Here's how the part is built. I have some questions about the finished solid (model axes, mm). A direction names the side the tool comes from. Give positions to 0.01 mm unless a question says otherwise; leave off trailing zeros. Write each loop counter-clockwise with the first axis right and the second up, starting at its lowest first coordinate (ties: lowest second). Pieces come first, ordered by that corner, then holes. Notation, with made-up numbers: (58, 0) -> (107, 0) arc R16 cw to (107, 17) -> close; hole circle Ø2 at (-17.75, 87). An arc over 180 degrees is marked (long way). Use one line per item in the form item = value.
```python
from build123d import *

# Parameters (mm, degrees)
EXTRUDE_1_DEPTH           = 5
HOLE_WIZARD_M5_1_D        = 5.3
CUT_EXTRUDE_1_DEPTH       = 2.5
HOLE_WIZARD_2_0_2_1_D     = 2
HOLE_WIZARD_2_0_2_1_DEPTH = 5
HOLE_WIZARD_2_0_2_2_D     = 2
HOLE_WIZARD_2_0_2_2_DEPTH = 55
HOLE_WIZARD_M5_2_D        = 5.3
HOLE_WIZARD_M5_2_DEPTH    = 12.4


with BuildPart() as part:
    # 스케치1 → 보스-돌출1 (new, symmetric)
    with BuildSketch(Plane.XY):
        with BuildLine():
            Line((-32, 0), (32, 0))
            Line((32, 0), (32, 6))
            Line((32, 6), (16.781610859, 57.462613925))
            ThreePointArc((16.781610859, 57.462613925), (0, 70), (-16.781610859, 57.462613925))
            Line((-16.781610859, 57.462613925), (-32, 6))
            Line((-32, 6), (-32, 0))
        make_face()
    extrude(amount=EXTRUDE_1_DEPTH, both=True)

    # M5 여유 구멍1 (through all)
    with Locations(Plane.XY.offset(5)):
        with Locations((0, 53)):
            Hole(HOLE_WIZARD_M5_1_D / 2)

    # 스케치4 → 컷-돌출1 (cut)
    with BuildSketch(Plane.XY.offset(5)):
        with BuildLine():
            ThreePointArc((-10.585585486, 60.184777453), (-12.793578355, 53), (-10.585585486, 45.815222547))
            ThreePointArc((-10.585585486, 45.815222547), (-6.418566116, 45.017758083), (-5.621101652, 49.184777453))
            ThreePointArc((-5.621101652, 49.184777453), (-6.793578355, 53), (-5.621101652, 56.815222547))
            ThreePointArc((-5.621101652, 56.815222547), (-6.418566116, 60.982241917), (-10.585585486, 60.184777453))
        make_face()
    cut_extrude_1 = extrude(amount=-CUT_EXTRUDE_1_DEPTH, mode=Mode.SUBTRACT)

    # Ø2.0 (2) 지름 구멍1
    with Locations(Plane.XY.offset(5)):
        with Locations((-8, 53)):
            hole_wizard_2_0_2_1 = Hole(HOLE_WIZARD_2_0_2_1_D / 2, depth=HOLE_WIZARD_2_0_2_1_DEPTH)

    # 대칭 복사1: 컷-돌출1, Ø2.0 (2) 지름 구멍1 across plane
    add(cut_extrude_1.mirror(Plane(origin=(0, 0, 0), x_dir=(0, 0, 1), z_dir=(1, 0, 0))), mode=Mode.SUBTRACT)
    add(hole_wizard_2_0_2_1.mirror(Plane(origin=(0, 0, 0), x_dir=(0, 0, 1), z_dir=(1, 0, 0))), mode=Mode.SUBTRACT)

    # Ø2.0 (2) 지름 구멍2
    with Locations(Plane(origin=(0, 0, 0), x_dir=(-1, 0, 0), z_dir=(0, -1, 0))):
        with Locations((-8, 0), (8, 0)):
            Hole(HOLE_WIZARD_2_0_2_2_D / 2, depth=HOLE_WIZARD_2_0_2_2_DEPTH)

    # M5 여유 구멍2
    with Locations(Plane(origin=(0, 0, 0), x_dir=(-1, 0, 0), z_dir=(0, -1, 0))):
        with Locations((-22, 0), (22, 0)):
            Hole(HOLE_WIZARD_M5_2_D / 2, depth=HOLE_WIZARD_M5_2_DEPTH)


solid = part.part
```
Q1. I want a section at B-B, the plane y = 53. Write out the boundary of the cut face in (x, z).
Result set:
outline = (-18.1, -5) -> (-2.65, -5) -> (-2.65, 5) -> (-6.79, 5) -> (-6.79, 2.5) -> (-7, 2.5) -> (-7, 0) arc R1 cw to (-9, 0) -> (-9, 2.5) -> (-12.79, 2.5) -> (-12.79, 5) -> (-18.1, 5) -> close; (2.65, -5) -> (18.1, -5) -> (18.1, 5) -> (12.79, 5) -> (12.79, 2.5) -> (9, 2.5) -> (9, 0) arc R1 cw to (7, 0) -> (7, 2.5) -> (6.79, 2.5) -> (6.79, 5) -> (2.65, 5) -> close
Q2. I want a section at A-A, the plane x = 0. Write out the boundary of the cut face in (y, z).
Result set:
outline = (0, -5) -> (50.35, -5) -> (50.35, 5) -> (0, 5) -> close; (55.65, -5) -> (70, -5) -> (70, 5) -> (55.65, 5) -> close
Q3. Which directions (+Z, -Z, +X, -X, +Y, -Y) give clear straight access to the entire face, cutting with the end or side of a thin tool? Please do faces 4 (the face through (24.528, 6.287, -0.796)), 5 (the face through (0.34, 55.63, -0.07)), 6 (the face through (7, 53, 2)).
Result set:
face_4 = -Y
face_5 = +Z, -Z
face_6 = +Z
Q4. If I drill on line 1 along Z through (x, y) = (-8, 24.5); line 2 along X through (y, z) = (17, 0.5); line 3 along Z through (x, y) = (22, 8), over which ranges is the centre line in solid material (lowest first)? Write a range as from..to.
Result set:
line_1 = -5..-1, 1..5
line_2 = -28.75..-8.87, -7.13..7.13, 8.87..28.75
line_3 = -5..-2.65, 2.65..5
Q5. Will these pins go through, and if not, where does the flat tip stop? pin 1 Ø1 at (x, z) = (21, 1) entering from -Y; pin 2 Ø5 at (x, z) = (12, -1.5) entering from -Y; pin 3 Ø1.2 at (x, y) = (-8, 53) entering from +Z; pin 4 Ø2.5 at (x, z) = (-8, 0) entering from +Y.
Result set:
pin_1 = 12.4
pin_2 = 0
pin_3 = -0.8
pin_4 = 68.65
Q6. I want a section at D-D, the plane x = 22. Write out the boundary of the cut face in (y, z).
Result set:
outline = (0, -5) -> (39.82, -5) -> (39.82, 5) -> (0, 5) -> (0, 2.65) -> (12.4, 2.65) -> (12.4, -2.65) -> (0, -2.65) -> close
Q7. I want a section at C-C, the plane y = 15. Write out the boundary of the cut face in (x, z).
Result set:
outline = (-29.34, -5) -> (29.34, -5) -> (29.34, 5) -> (-29.34, 5) -> close; hole circle Ø2 at (-8, 0); hole circle Ø2 at (8, 0)
Q8. If we mould it in two halves opening along Y, with no side actions, what happens to faces 1 (the face through (12.793, 53.107, 3.768)), 2 (the face through (8, 55, 0)), 3 (the face through (-32, 3, 0))? For each: +Y half, -Y half, draft (parallel to the pull), parting line (faces both ways), or undercut.
Result set:
face_1 = undercut
face_2 = -Y half
face_3 = draft
